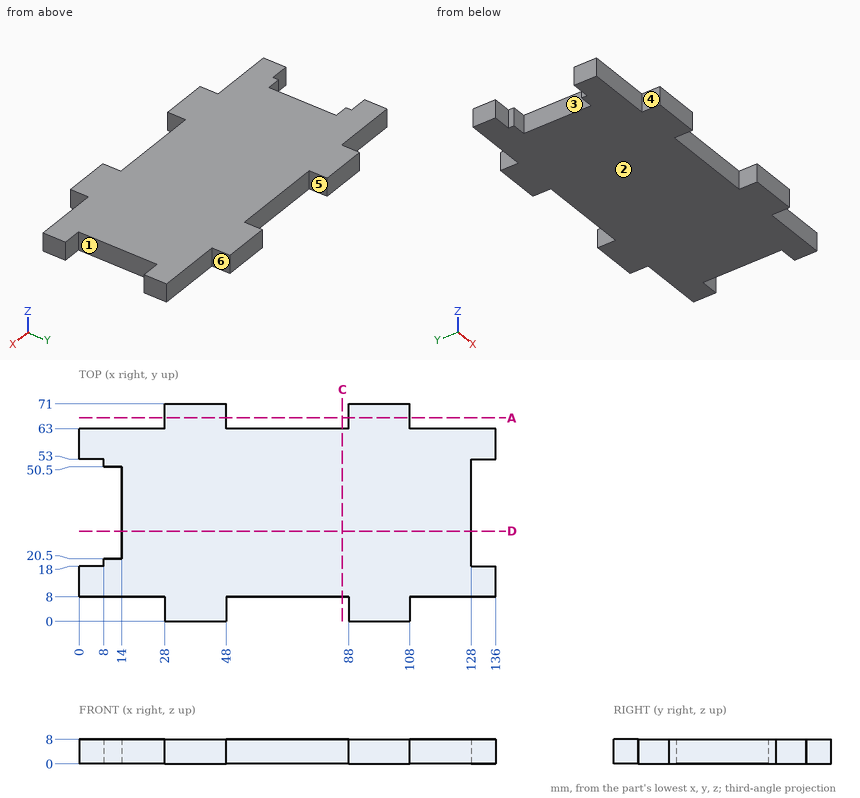
For this review, use the dimensioned drawing (mm, ordinates from the lowest corner) and the shaded views. A direction names the side the tool comes from. Coordinates: 2 decimals unless noted, no trailing zeros. Order: outer loops, then holes, each group sorted by start corner. A loop starts at its lowest first (then second) coordinate and runs counter-clockwise, first axis right, second up. Notation, with made-up numbers: (87.25, 83) - (132.25, 83) arc R12 ccw to (132.25, 94) - close; hole circle Ø11 at (45, -4). An arc over 180 degrees is marked (long way). Answer as a JSON object with one key per item and string values. Group by question number.
1. We need section A-A on y = 66.5. State the section outline as (x, z) points, then the cut area to 3 significant figures.
2. We need section C-C on x = 86. State the section outline as (y, z) points, then the cut area to 3 significant figures.
3. We need section D-D on y = 29.5. State the section outline as (x, z) points.
4. The part is to be moulded in two halves that separate along Y. For the marked faces 1 and 2, say which applies: pulls with the +Y half, pulls with the -Y half, needs draft (parallel to the pull), parting line crosses it, or undercut.
5. For the marked faces 3, 4, 5 and 6, list the 3-axis set-ups (+Z, -Z, +X, -X, +Y, -Y) from which the entire face can be reached by the end or side of a thin tool; tool diameter is ignored.
6. For probe 1 along Y at (x, z) = (6, 6.25); probe 2 along X at (y, z) = (66, 0.5); probe 3 along Y at (x, z) = (120.5, 4.5), list the stretches that pass through material, from the lowest coordinate up.
7. Clearance check with flat-ended pins moving along their axes: P1, Ø1, axis at x = 73.5, z = 2.5, coming from the -Y side; P2, Ø4, axis at x = 24, z = 4, coming from the +Y side; P3, Ø2.5, axis at y = 2, z = 4, coming from the +X side. State where each tip first meets the part, or that it passes through.
Final values:
{
 "1": {"outline": "(28, 0) - (48, 0) - (48, 8) - (28, 8) - close; (88, 0) - (108, 0) - (108, 8) - (88, 8) - close", "area": "320 mm²"},
 "2": {"outline": "(8, 0) - (63, 0) - (63, 8) - (8, 8) - close", "area": "440 mm²"},
 "3": {"outline": "(14, 0) - (128, 0) - (128, 8) - (14, 8) - close"},
 "4": {"face 1": "undercut", "face 2": "needs draft"},
 "5": {"face 3": "+Z, -Z, -X", "face 4": "+Z, -Z, -X, -Y", "face 5": "+Z, -Z, +Y", "face 6": "+Z, -Z, +X, +Y"},
 "6": {"probe 1": "8 to 18, 53 to 63", "probe 2": "28 to 48, 88 to 108", "probe 3": "8 to 63"},
 "7": {"P1": "y = 8", "P2": "y = 63", "P3": "x = 108"}
}
